from build123d import *

# Parameters (mm, degrees)
SKETCH1_W           = 26
SKETCH1_H           = 40
SKETCH1_W_2         = 6
SKETCH1_H_2         = 3
BOSS_EXTRUDE1_DEPTH = 1.2
SKETCH2_W           = 26
SKETCH2_H           = 40
SKETCH2_W_2         = 16
SKETCH2_H_2         = 16
BOSS_EXTRUDE2_DEPTH = 1.3
SKETCH5_W           = 26
SKETCH5_H           = 40
SKETCH5_W_2         = 23.6
SKETCH5_H_2         = 37.6
BOSS_EXTRUDE3_DEPTH = 8
SKETCH6_R           = 2
CUT_EXTRUDE1_DEPTH  = 8


with BuildPart() as part:
    # Sketch1 → Boss-Extrude1 (new body)
    with BuildSketch(Plane.XY):
        with Locations((8, -8)):
            Rectangle(SKETCH1_W, SKETCH1_H)
        with Locations((8, -8)):
            Rectangle(SKETCH1_W_2, SKETCH1_H_2, mode=Mode.SUBTRACT)
    extrude(amount=BOSS_EXTRUDE1_DEPTH)

    # Sketch2 → Boss-Extrude2 (add)
    with BuildSketch(Plane(origin=(0, 0, 0), x_dir=(-1, 0, 0), z_dir=(0, 0, -1))):
        with Locations((-8, -8)):
            Rectangle(SKETCH2_W, SKETCH2_H)
        with Locations((-8, -8)):
            Rectangle(SKETCH2_W_2, SKETCH2_H_2, mode=Mode.SUBTRACT)
    extrude(amount=BOSS_EXTRUDE2_DEPTH)

    # Sketch5 → Boss-Extrude3 (add)
    with BuildSketch(Plane(origin=(0, 0, -1.3), x_dir=(-1, 0, 0), z_dir=(0, 0, -1))):
        with Locations((-8, -8)):
            Rectangle(SKETCH5_W, SKETCH5_H)
        with Locations((-8, -8)):
            Rectangle(SKETCH5_W_2, SKETCH5_H_2, mode=Mode.SUBTRACT)
    extrude(amount=BOSS_EXTRUDE3_DEPTH)

    # Sketch6 → Cut-Extrude1 (cut)
    with BuildSketch(Plane.XZ.offset(28)):
        with Locations(Location((8, -4.05, 0), (0, 0, 270))):
            Circle(SKETCH6_R)
    extrude(amount=-CUT_EXTRUDE1_DEPTH, mode=Mode.SUBTRACT)


solid = part.part
Part model, mm, in its own coordinate system. A direction names the side the tool comes from. Coordinates: 2 decimals unless noted, no trailing zeros. Write each loop counter-clockwise with the first axis right and the second up, starting at its lowest first coordinate (ties: lowest second). Pieces come first, ordered by that corner, then holes. Notation, with made-up numbers: M -5.75,-29 L 52.25,-29 A17 cw 52.25,-9 Z; hole C -10.5,84.5 d8. An arc over 180 degrees is marked long. Return JSON: item names as keys, results as strings.
1. Saw through at C-C, the plane y = -15. Write the cut outline in (x, z), then the cut area to 3 significant figures.
Determined:
{"outline": "M -5,-9.3 L -3.8,-9.3 L -3.8,-1.3 L 0,-1.3 L 0,0 L 16,0 L 16,-1.3 L 19.8,-1.3 L 19.8,-9.3 L 21,-9.3 L 21,1.2 L -5,1.2 Z", "area": "63.4 mm²"}
2. Pull direction Y, two halves, no side cores. Call faces 1 (the face through (8, -12, 1.2)), 2 (the face through (8, 12, -4)), 3 (the face through (8.2, -28, -6.3)), 4 (the face through (16, -8, -1)): pulls with the +Y half, pulls with the -Y half, needs draft (parallel to the pull), parting line crosses it, or undercut.
Determined:
{"face 1": "needs draft", "face 2": "pulls with the +Y half", "face 3": "pulls with the -Y half", "face 4": "undercut"}
3. Flat gauge pins, fed straight in: pin 1 Ø2.5 at (x, z) = (7.5, -5.5) entering from -Y; pin 2 Ø4 at (x, y) = (2.5, -8.5) entering from -Z; pin 3 Ø13 at (x, y) = (9, -6) entering from -Z. Where does each tip first touch, or does it go through?
Determined:
{"pin 1": "y = -28", "pin 2": "z = 0", "pin 3": "z = -1.3"}
4. Probe L1, parallel to X at y = -27.1, z = -4.05; L2, parallel to X at y = -13.5, z = -2.5; L3, parallel to Y at x = 12.5, z = -5. List the from-to ranges inside material, lowest first.
Determined:
{"L1": "-5 to 6, 10 to 21", "L2": "-5 to -3.8, 19.8 to 21", "L3": "-28 to -26.8, 10.8 to 12"}
5. 3-axis set-ups, long thin cutter, end or side, ignore diameter. For faces 5 (the face through (8, -6.5, 1)), 6 (the face through (8, -26.8, -7)), 7 (the face through (8.601, -27.408, -5.958)), 8 (the face through (21, -8, -4)), 9 (the face through (20.6, -7.9, -9.3)): which of +Z, -Z, +X, -X, +Y, -Y reach the whole face in a straight line?
Determined:
{"face 5": "+Z, -Z", "face 6": "-Z", "face 7": "-Y", "face 8": "+Z, -Z, +X, +Y, -Y", "face 9": "-Z, +X, -X, +Y, -Y"}
6. Saw through at D-D, the plane x = 17.5. Write the cut outline in (y, z).
Determined:
{"outline": "M -28,-9.3 L -26.8,-9.3 L -26.8,-1.3 L 10.8,-1.3 L 10.8,-9.3 L 12,-9.3 L 12,1.2 L -28,1.2 Z"}
7. Saw through at A-A, the plane z = -7. Write the cut outline in (x, y), then the cut area to 3 significant figures.
Determined:
{"outline": "M -5,-28 L 21,-28 L 21,12 L -5,12 Z; hole M -3.8,-26.8 L 19.8,-26.8 L 19.8,10.8 L -3.8,10.8 Z", "area": "153 mm²"}
8. Saw through at B-B, the plane x = 8. Write the cut outline in (y, z), then the cut area to 3 significant figures.
Determined:
{"outline": "M -28,-9.3 L -26.8,-9.3 L -26.8,-6.05 L -28,-6.05 Z; M -28,-2.05 L -26.8,-2.05 L -26.8,-1.3 L -16,-1.3 L -16,0 L -9.5,0 L -9.5,1.2 L -28,1.2 Z; M -6.5,0 L 0,0 L 0,-1.3 L 10.8,-1.3 L 10.8,-9.3 L 12,-9.3 L 12,1.2 L -6.5,1.2 Z", "area": "90.0 mm²"}
